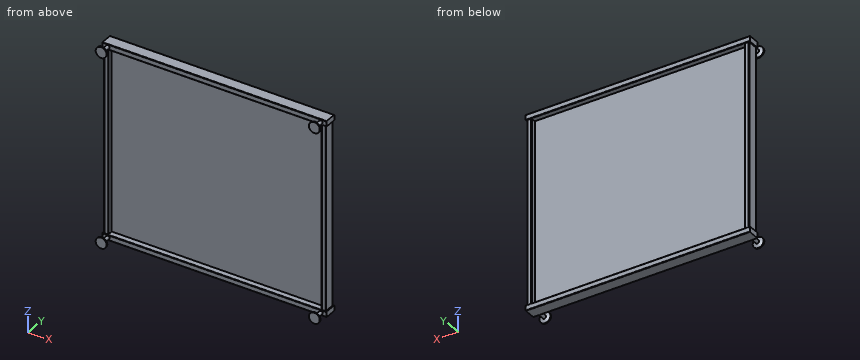
```python
from build123d import *

# Parameters (mm, degrees)
EXTRUDE_1_DEPTH      = 425
EXTRUDE_1_2_DEPTH    = 425
EXTRUDE_4_DEPTH      = 515
EXTRUDE_4_DEPTH_BACK = 515
SKETCH_3_W           = 980
SKETCH_3_H           = 850
EXTRUDE_5_DEPTH      = 2


with BuildPart() as part:
    # Sketch 1 → Extrude 1 (new, symmetric)
    with BuildSketch(Plane.XY):
        with BuildLine():
            Line((-507, 25), (-493, 25))
            ThreePointArc((-493, 25), (-490.878679656, 24.121320344), (-490, 22))
            Line((-490, 22), (-490, -22))
            ThreePointArc((-490, -22), (-490.878679656, -24.121320344), (-493, -25))
            Line((-493, -25), (-507, -25))
            ThreePointArc((-507, -25), (-509.121320344, -24.121320344), (-510, -22))
            Line((-510, -22), (-510, 22))
            ThreePointArc((-510, 22), (-509.121320344, 24.121320344), (-507, 25))
        make_face()
        with BuildLine():
            Line((-508.5, 22), (-508.5, -22))
            ThreePointArc((-508.5, -22), (-508.060660172, -23.060660172), (-507, -23.5))
            Line((-507, -23.5), (-493, -23.5))
            ThreePointArc((-493, -23.5), (-491.939339828, -23.060660172), (-491.5, -22))
            Line((-491.5, -22), (-491.5, 22))
            ThreePointArc((-491.5, 22), (-491.939339828, 23.060660172), (-493, 23.5))
            Line((-493, 23.5), (-507, 23.5))
            ThreePointArc((-507, 23.5), (-508.060660172, 23.060660172), (-508.5, 22))
        make_face(mode=Mode.SUBTRACT)
    extrude(amount=EXTRUDE_1_DEPTH, both=True)



with BuildPart() as body_2:
    # Sketch 1 → Extrude 1 2 (new, symmetric)
    with BuildSketch(Plane.XY):
        with BuildLine():
            Line((490, 22), (490, -22))
            ThreePointArc((490, -22), (490.878679656, -24.121320344), (493, -25))
            Line((493, -25), (507, -25))
            ThreePointArc((507, -25), (509.121320344, -24.121320344), (510, -22))
            Line((510, -22), (510, 22))
            ThreePointArc((510, 22), (509.121320344, 24.121320344), (507, 25))
            Line((507, 25), (493, 25))
            ThreePointArc((493, 25), (490.878679656, 24.121320344), (490, 22))
        make_face()
        with BuildLine():
            Line((507, 23.5), (493, 23.5))
            ThreePointArc((493, 23.5), (491.939339828, 23.060660172), (491.5, 22))
            Line((491.5, 22), (491.5, -22))
            ThreePointArc((491.5, -22), (491.939339828, -23.060660172), (493, -23.5))
            Line((493, -23.5), (507, -23.5))
            ThreePointArc((507, -23.5), (508.060660172, -23.060660172), (508.5, -22))
            Line((508.5, -22), (508.5, 22))
            ThreePointArc((508.5, 22), (508.060660172, 23.060660172), (507, 23.5))
        make_face(mode=Mode.SUBTRACT)
    extrude(amount=EXTRUDE_1_2_DEPTH, both=True)

    # Sketch 2 → Extrude 4 (add, two sides: drawn at the far end of the back side and taken through both)
    with BuildSketch(Plane(origin=(0, 0, 0), x_dir=(0, 0, -1), z_dir=(1, 0, 0)).offset(-EXTRUDE_4_DEPTH_BACK)):
        with BuildLine():
            Line((425, -25), (425, 25))
            ThreePointArc((425, 25), (425.878679656, 27.121320344), (428, 28))
            Line((428, 28), (447, 28))
            ThreePointArc((447, 28), (449.121320344, 27.121320344), (450, 25))
            Line((450, 25), (450, -25))
            ThreePointArc((450, -25), (449.121320344, -27.121320344), (447, -28))
            Line((447, -28), (428, -28))
            ThreePointArc((428, -28), (425.878679656, -27.121320344), (425, -25))
        make_face()
        with BuildLine():
            Line((-428, -28), (-447, -28))
            ThreePointArc((-447, -28), (-449.121320344, -27.121320344), (-450, -25))
            Line((-450, -25), (-450, 25))
            ThreePointArc((-450, 25), (-449.121320344, 27.121320344), (-447, 28))
            Line((-447, 28), (-428, 28))
            ThreePointArc((-428, 28), (-425.878679656, 27.121320344), (-425, 25))
            Line((-425, 25), (-425, -25))
            ThreePointArc((-425, -25), (-425.878679656, -27.121320344), (-428, -28))
        make_face()
    extrude(amount=EXTRUDE_4_DEPTH + EXTRUDE_4_DEPTH_BACK)


with BuildPart() as part_1:
    add(part.part)

    add(body_2.part)  # Extrude 5 merges body 2
    # Sketch 3 → Extrude 5 (add)
    with BuildSketch(Plane(origin=(0, 0, 0), x_dir=(1, 0, 0), z_dir=(0, 1, 0))):
        Rectangle(SKETCH_3_W, SKETCH_3_H)
    extrude(amount=EXTRUDE_5_DEPTH)

    # Sketch 4 → Revolve 1 (revolve)
    with BuildSketch(Plane(origin=(-490, 0, 0), x_dir=(0, 0, -1), z_dir=(1, 0, 0)), mode=Mode.PRIVATE) as revolve_1_sk:
        Polygon((-437.5, -28), (-429.5, -28), (-429.5, -65), (-427.5, -65), (-412.5, -70), (-412.5, -75), (-437.5, -75), align=None)
    revolve_1 = revolve(revolve_1_sk.sketch.rotate(Axis((-490, 28, 437.5), (0, -1, 0)), 180), axis=Axis((-490, 28, 437.5), (0, -1, 0)))

    # Mirror 1: Revolve 1 across plane
    add(revolve_1.mirror(Plane(origin=(0, 0, 0), x_dir=(0, 0, 1), z_dir=(1, 0, 0))))

    # Mirror 2: Revolve 1 across plane
    add(revolve_1.mirror(Plane.XY))

    # Mirror 2 copy 1 sketch → Mirror 2 copy 1 (revolve)
    with BuildSketch(Plane.ZY.offset(-490)):
        Polygon((-437.5, -28), (-429.5, -28), (-429.5, -65), (-427.5, -65), (-412.5, -70), (-412.5, -75), (-437.5, -75), align=None)
    revolve(axis=Axis((490, 28, -437.5), (0, -1, 0)))


solid = part_1.part
```
For this review, take the finished solid that the model builds, in its own axes (mm). Give positions to 0.01 mm unless a question says otherwise; leave off trailing zeros. Order: outer loops, then holes, each group sorted by start corner. A loop starts at its lowest first (then second) coordinate and runs counter-clockwise, first axis right, second up.
1) Insertion check: pin 1 (13 mm diameter, centred on y = -8, z = 27.5, fed in from -X); pin 2 (7 mm diameter, centred on x = -497, z = 149, fed in from -Y); pin 3 (21 mm diameter, centred on x = -132.5, z = 437, fed in from -Y). Each pin has a flat end and moves straight along its axis. Give the tip position at first contact, or say it passes through.
2) Wall thickness on line 1 (X direction, y = 14, z = -252.5); line 2 (X direction, y = 1.5, z = 381); line 3 (Z direction, x = 255, y = -23): over which ranges is each line inside the solid? List them lowest first.
3) Take a section at A-A (x = -91). Give the boundary of the cut face in (y, z).
4) Take a section at B-B (z = -240). State how many separate pieces and enclosed holes the cut face has, then the cut area to 3 significant figures.
Derived:
1. pin 1: stops at x = -510
1. pin 2: stops at y = -25
1. pin 3: stops at y = -28
2. line 1: x = -510 to -508.5, -491.5 to -490, 490 to 491.5, 508.5 to 510
2. line 2: x = -510 to -508.5, -491.5 to 491.5, 508.5 to 510
2. line 3: z = -450 to -425, 425 to 450
3. outline: (-28, -447) arc R3 ccw to (-25, -450) - (25, -450) arc R3 ccw to (28, -447) - (28, -428) arc R3 ccw to (25, -425) - (2, -425) - (2, 425) - (25, 425) arc R3 ccw to (28, 428) - (28, 447) arc R3 ccw to (25, 450) - (-25, 450) arc R3 ccw to (-28, 447) - (-28, 428) arc R3 ccw to (-25, 425) - (0, 425) - (0, -425) - (-25, -425) arc R3 ccw to (-28, -428) - close
4. separate pieces: 1
4. enclosed holes: 2
4. area: 2,350 mm2
